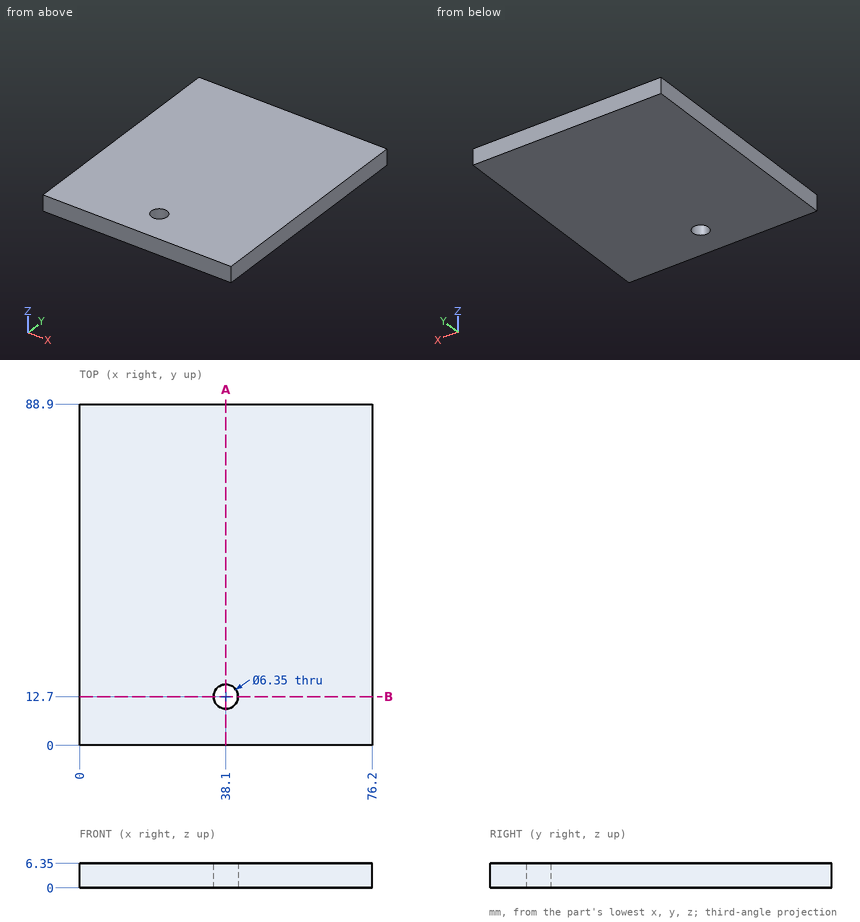
Study the drawing (mm; zero at the part's minimum x, y, z) and answer. Give positions to 0.01 mm unless a question says otherwise; leave off trailing zeros. Order: outer loops, then holes, each group sorted by start corner. A loop starts at its lowest first (then second) coordinate and runs counter-clockwise, first axis right, second up. Notation, with made-up numbers: (64.25, 44.5) - (97.25, 44.5) arc R26 ccw to (97.25, 74.5) - close; hole circle Ø3 at (-1, 7.25). An arc over 180 degrees is marked (long way). Answer in a Markdown table with one row per item. Add a question column.
Q1. The part is cut by section B-B (y = 12.7). Determine the outline of the cut face in (x, z) (3 decimals).
Q2. Given P1, Ø5, axis at x = 64.5, y = 21, coming from the -Z side; P2, Ø5.5, axis at x = 38.1, y = 12.7, coming from the +Z side, each flat-ended and moving along its own axis, determine where each tip first touches the part or whether it passes through.
Q3. Find the intervals of material crossed by line 1 along Y through (x, z) = (38.1, 2) (3 decimals); line 2 along X through (y, z) = (12.7, 4.5) (3 decimals); line 3 along X through (y, z) = (13.5, 2), in increasing order. Write a range as [from, to].
Q4. The part is cut by section A-A (x = 38.1). Determine the outline of the cut face in (y, z) (3 decimals), then the cut area to 3 significant figures.
Determined:
| question | item | result |
|---|---|---|
| 1 | outline | (0, 0) - (34.925, 0) - (34.925, 6.35) - (0, 6.35) - close; (41.275, 0) - (76.2, 0) - (76.2, 6.35) - (41.275, 6.35) - close |
| 2 | P1 | stops at z = 0 |
| 2 | P2 | passes through |
| 3 | line 1 | y = [0, 9.525], [15.875, 88.9] |
| 3 | line 2 | x = [0, 34.925], [41.275, 76.2] |
| 3 | line 3 | x = [0, 35.03], [41.17, 76.2] |
| 4 | outline | (0, 0) - (9.525, 0) - (9.525, 6.35) - (0, 6.35) - close; (15.875, 0) - (88.9, 0) - (88.9, 6.35) - (15.875, 6.35) - close |
| 4 | area | 524 mm² |
